```python
from build123d import *

# Parameters (mm, degrees)
SKETCH1_W           = 22
SKETCH1_H           = 12
BOSS_EXTRUDE1_DEPTH = 22
SKETCH2_W           = 32
SKETCH2_H           = 2
BOSS_EXTRUDE2_DEPTH = 12
SKETCH3_R           = 1
CUT_EXTRUDE1_DEPTH  = 22
SKETCH5_R           = 6
BOSS_EXTRUDE3_DEPTH = 5
SKETCH6_R           = 2.5
BOSS_EXTRUDE4_DEPTH = 3


with BuildPart() as part:
    # Sketch1 → Boss-Extrude1 (new body)
    with BuildSketch(Plane(origin=(0, 0, 0), x_dir=(1, 0, 0), z_dir=(0, 1, 0))):
        with Locations((11, 6)):
            Rectangle(SKETCH1_W, SKETCH1_H)
    extrude(amount=BOSS_EXTRUDE1_DEPTH)

    # Sketch2 → Boss-Extrude2 (add, through all)
    with BuildSketch(Plane.XY):
        with Locations((11, 17)):
            Rectangle(SKETCH2_W, SKETCH2_H)
    extrude(amount=-BOSS_EXTRUDE2_DEPTH)

    # Sketch3 → Cut-Extrude1 (cut)
    with BuildSketch(Plane(origin=(0, 18, 0), x_dir=(1, 0, 0), z_dir=(0, 1, 0))):
        with Locations(Location((-2.5, 6, 0), (0, 0, 270))):
            Circle(SKETCH3_R)
        with Locations(Location((24.5, 6, 0), (0, 0, 270))):
            Circle(SKETCH3_R)
    extrude(amount=-CUT_EXTRUDE1_DEPTH, mode=Mode.SUBTRACT)

    # Sketch5 → Boss-Extrude3 (add)
    with BuildSketch(Plane(origin=(0, 22, 0), x_dir=(1, 0, 0), z_dir=(0, 1, 0))):
        with Locations(Location((16, 6, 0), (0, 0, 270))):
            Circle(SKETCH5_R)
    extrude(amount=BOSS_EXTRUDE3_DEPTH)

    # Sketch6 → Boss-Extrude4 (add)
    with BuildSketch(Plane(origin=(0, 27, 0), x_dir=(1, 0, 0), z_dir=(0, 1, 0))):
        with Locations(Location((16, 6, 0), (0, 0, 270))):
            Circle(SKETCH6_R)
    extrude(amount=BOSS_EXTRUDE4_DEPTH)


solid = part.part
```
The listing builds one solid part. Answer for the finished solid, in the listing's coordinates (mm). A direction names the side the tool comes from. Give positions to 0.01 mm unless a question says otherwise; leave off trailing zeros. Order: outer loops, then holes, each group sorted by start corner. A loop starts at its lowest first (then second) coordinate and runs counter-clockwise, first axis right, second up. Notation, with made-up numbers: (18, 37.25) - (54, 37.25) arc R19 cw to (54, 44.25) - close; hole circle Ø6 at (-17, 38.25). An arc over 180 degrees is marked (long way). Use one line per item in the form item = value. Start each with the question number.
(1) A cutting plane is placed at A-A, the plane x = -2.5. Write down the section's boundary in (y, z), then the cut area to 3 significant figures.
(2) A cutting plane is placed at C-C, the plane y = 23. Write down the section's boundary in (x, z).
(3) For faces 5 (the cylindrical face through (15.04, 28.48, -3.69)), 6 (the flat face through (26, 16, -6)), 7 (the flat face through (0, 8, -6)), 8 (the flat face through (26, 18, -6)), 9 (the flat face through (-1, 18, -6)), determine the directions among +Z, -Z, +X, -X, +Y, -Y from which every point of the face is accessible in a straight line to the end or side of a thin tool.
(4) A cutting plane is placed at D-D, the plane z = -9. Write down the section's boundary in (x, y).
(5) Consider line 1 (X direction, y = 16.7, z = -6); line 2 (Y direction, x = 9, z = -5). Determine where each line is inside the solid, lowest interval first. Write a range as from..to.
(6) A cutting plane is placed at B-B, the plane z = -5.5. State how many separate pieces and enclosed holes the cut face has, then the cut area to 3 significant figures.
(7) The mould has two halves that part along X. Classify faces 1 (the flat face through (16, 30, -6)), 2 (the cylindrical face through (-3.1, 17, -6.8)), 3 (the cylindrical face through (23.524, 17.014, -6.217)), 4 (the flat face through (22, 20, -6)): released by +X, released by -X, zero draft, split by the parting line, or undercut.
(8) Flat-ended cylindrical pins translate along their axes: pin 1 Ø1.2 at (y, z) = (20, -8.5) entering from +X; pin 2 Ø1.2 at (x, z) = (24.5, -6) entering from +Y; pin 3 Ø1.2 at (y, z) = (21, -3) entering from -X; pin 4 Ø1.5 at (x, z) = (-2, -6.5) entering from +Y. Find the tip coordinate at first contact, or state that the pin passes through.
Ans:
q1.outline = (16, -12) - (18, -12) - (18, -7) - (16, -7) - close; (16, -5) - (18, -5) - (18, 0) - (16, 0) - close
q1.area = 20.0 mm^2
q2.outline = circle Ø12 at (16, -6)
q3.face_5 = +Y
q3.face_6 = +Z, -Z, +X, -Y
q3.face_7 = +Z, -Z, -X, -Y
q3.face_8 = +Z, -Z, +X, +Y
q3.face_9 = +Z, -Z, -X, +Y
q4.outline = (-5, 16) - (0, 16) - (0, 0) - (22, 0) - (22, 16) - (27, 16) - (27, 18) - (22, 18) - (22, 22) - (21.2, 22) - (21.2, 27) - (10.8, 27) - (10.8, 22) - (0, 22) - (0, 18) - (-5, 18) - close
q5.line_1 = -5..-3.5, -1.5..23.5, 25.5..27
q5.line_2 = 0..22
q6.separate_pieces = 3
q6.enclosed_holes = 0
q6.area = 572 mm^2
q7.face_1 = zero draft
q7.face_2 = undercut
q7.face_3 = undercut
q7.face_4 = released by +X
q8.pin_1 = 22
q8.pin_2 = through
q8.pin_3 = 0
q8.pin_4 = 18
